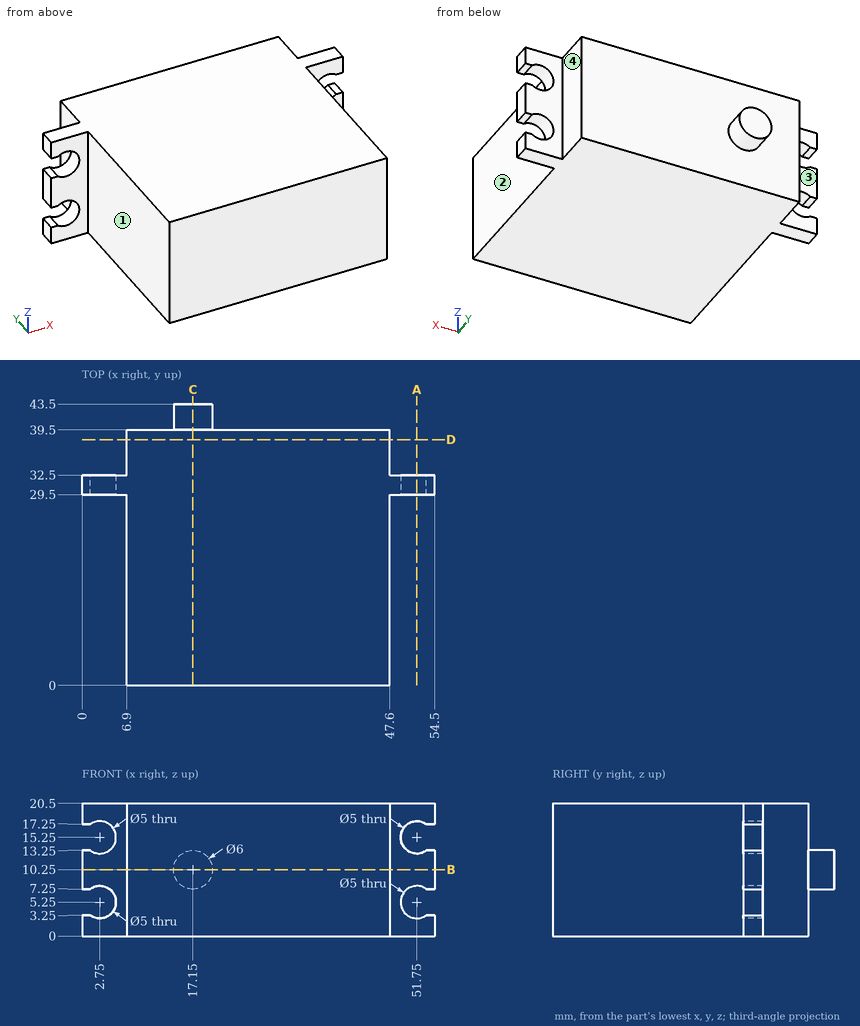
Verification items for this drawing (mm, ordinates from the low corner). A direction names the side the tool comes from. Give positions to 0.01 mm unless a question says otherwise; leave off trailing zeros. Write each loop counter-clockwise with the first axis right and the second up, starting at its lowest first coordinate (ties: lowest second). Pieces come first, ordered by that corner, then holes. Notation, with made-up numbers: (-5.75, 9.5) -> (14.25, 9.5) arc R18 cw to (14.25, 13.5) -> close; hole circle Ø9 at (77, -28.5). An arc over 180 degrees is marked (long way). Use one line per item in the form item = value.
Item 1: Depth check by flat-ended pin: pin 1 Ø10 at (y, z) = (8, 8.5) entering from +X; pin 2 Ø10 at (y, z) = (15, 8) entering from -X; pin 3 Ø8 at (x, z) = (2.75, 15.25) entering from +Y. Enter the tip coordinate at first touch or a pass-through.
Results list:
pin_1 = 47.6
pin_2 = 6.9
pin_3 = 32.5
Item 2: Sectioned sample at D-D on y = 38. Enter the section's corners in (x, z).
Results list:
outline = (6.9, 0) -> (47.6, 0) -> (47.6, 20.5) -> (6.9, 20.5) -> close
Item 3: Access from +Z, -Z, +X, -X, +Y, -Y to the whole of each face (thin tool, end or side, straight path). Record for the marked faces 1, 2, 3 and 4.
Results list:
face_1 = +Z, -Z, -X, -Y
face_2 = +Z, -Z, +X, -Y
face_3 = +Z, -Z, -X, +Y
face_4 = +Z, -Z, +X, +Y
Item 4: Sectioned sample at C-C on x = 17.15. Enter the section's corners in (y, z).
Results list:
outline = (0, 0) -> (39.5, 0) -> (39.5, 7.25) -> (43.5, 7.25) -> (43.5, 13.25) -> (39.5, 13.25) -> (39.5, 20.5) -> (0, 20.5) -> close
Item 5: Scan lines: line 1 (Z direction, x = 51.75, y = 31.6); line 2 (Y direction, x = 35, z = 6.5); line 3 (X direction, y = 25, z = 12). Record each from-to range of solid material in increasing order.
Results list:
line_1 = 0 to 2.75, 7.75 to 12.75, 17.75 to 20.5
line_2 = 0 to 39.5
line_3 = 6.9 to 47.6
Item 6: Sectioned sample at B-B on z = 10.25. Enter the section's corners in (x, y).
Results list:
outline = (0, 29.5) -> (6.9, 29.5) -> (6.9, 0) -> (47.6, 0) -> (47.6, 29.5) -> (54.5, 29.5) -> (54.5, 32.5) -> (47.6, 32.5) -> (47.6, 39.5) -> (20.15, 39.5) -> (20.15, 43.5) -> (14.15, 43.5) -> (14.15, 39.5) -> (6.9, 39.5) -> (6.9, 32.5) -> (0, 32.5) -> close
Item 7: Sectioned sample at A-A on x = 51.75. Enter the section's corners in (y, z), plus the area to 3 significant figures.
Results list:
outline = (29.5, 0) -> (32.5, 0) -> (32.5, 2.75) -> (29.5, 2.75) -> close; (29.5, 7.75) -> (32.5, 7.75) -> (32.5, 12.75) -> (29.5, 12.75) -> close; (29.5, 17.75) -> (32.5, 17.75) -> (32.5, 20.5) -> (29.5, 20.5) -> close
area = 31.5 mm2
